Check sheet for the drawn part. Datum: minimum x, y, z corner. Units: mm. Round coordinates to 2 decimals unless told otherwise and drop trailing zeros. Write each loop counter-clockwise with the first axis right and the second up, starting at its lowest first coordinate (ties: lowest second). Pieces come first, ordered by that corner, then holes. Notation, with made-up numbers: (71, -39.75) - (107, -39.75) arc R18 ccw to (107, -15.75) - close; hole circle Ø6 at (54, 18.25). An arc over 180 degrees is marked (long way). Answer as a JSON object with one key per item and string values.
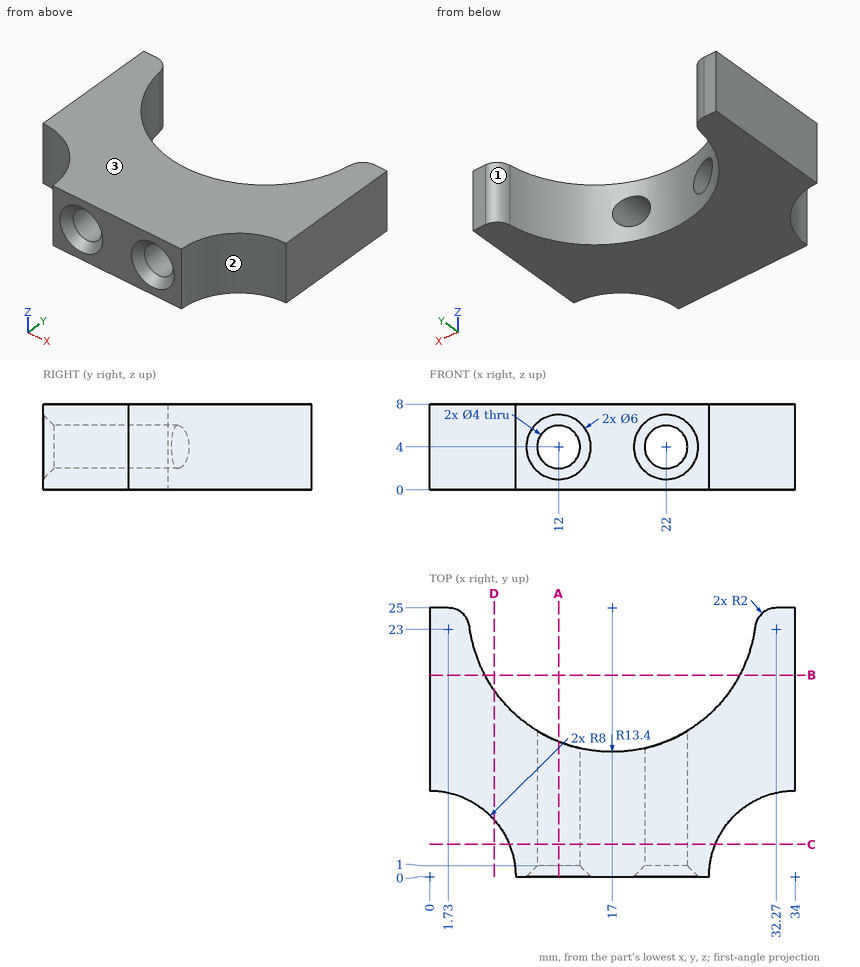
Q1. Material ranges on line 1 along X through (y, z) = (14.25, 6.25); line 2 along Z through (x, y) = (12, 9.25); line 3 along X through (y, z) = (3.5, 3) (1 decimal), recorded low to high. Write a range as [from, to].
Geometry check:
{"line 1": "x = [0, 9], [25, 34]", "line 2": "z = [0, 2], [6, 8]", "line 3": "x = [7.2, 10.3], [13.7, 20.3], [23.7, 26.8]"}
Q2. Section check C-C, the plane y = 3. Record the cut outline in (x, z), then the cut area to 3 significant figures.
Geometry check:
{"outline": "(7.42, 0) - (26.58, 0) - (26.58, 8) - (7.42, 8) - close; hole circle Ø4 at (12, 4); hole circle Ø4 at (22, 4)", "area": "128 mm2"}
Q3. Release check for a two-part mould opening along X. For the marked faces 1, 2 and 3 record: released by +X, released by -X, zero draft, split by the parting line, or undercut.
Geometry check:
{"face 1": "undercut", "face 2": "released by +X", "face 3": "zero draft"}
Q4. Section check A-A, the plane x = 12. Record the cut outline in (y, z).
Geometry check:
{"outline": "(0, 0) - (12.57, 0) - (12.57, 2) - (1, 2) - (0, 1) - close; (0, 7) - (1, 6) - (12.57, 6) - (12.57, 8) - (0, 8) - close"}
Q5. Gauge pin test, flat ends, axial feed: P1, Ø2, axis at x = 30, z = 4.5, coming from the +Y side (1 decimal); P2, Ø1, axis at x = 17, z = 1.5, coming from the +Y side; P3, Ø4.5, axis at x = 12, z = 4, coming from the -Y side. Record the tip position at first contact, or that the pin passes through.
Geometry check:
{"P1": "stops at y = 24.5", "P2": "stops at y = 11.61", "P3": "stops at y = 0.75"}
Q6. Section check B-B, the plane y = 18.75. Record the cut outline in (x, z).
Geometry check:
{"outline": "(0, 0) - (5.15, 0) - (5.15, 8) - (0, 8) - close; (28.85, 0) - (34, 0) - (34, 8) - (28.85, 8) - close"}
Q7. Section check D-D, the plane x = 6. Record the cut outline in (y, z).
Geometry check:
{"outline": "(5.29, 0) - (17.35, 0) - (17.35, 8) - (5.29, 8) - close"}
